Could you check a few things on this model? Use its own coordinates, in mm. A direction names the side the tool comes from. Round coordinates to 2 decimals unless told otherwise and drop trailing zeros. Loops run counter-clockwise (first coordinate to the right, second up) from the corner with the lowest first, then second, coordinate; pieces in that order, holes last. Notation, with made-up numbers: (20, 13.25) -> (51, 13.25) arc R13 cw to (51, 33.25) -> close; hole circle Ø6 at (79, 42.25). An arc over 180 degrees is marked (long way). One line per item, written item: value.
```python
from build123d import *

# Parameters (mm, degrees)
SKETCH1_R               = 3.75
BOSS_EXTRUDE1_DEPTH     = 10
SKETCH4_W               = 1
SKETCH4_H               = 1
BOSS_EXTRUDE2_DEPTH     = 2
CUT_EXTRUDE1_DEPTH      = 6.5
CUT_EXTRUDE1_DEPTH_BACK = 6.5
SKETCH5_W               = 3.094482754
SKETCH5_H               = 13.244386188
SKETCH6_R               = 3
BOSS_EXTRUDE3_DEPTH     = 6.7
SKETCH7_R               = 2.5
CUT_EXTRUDE2_DEPTH      = 1.25
FILLET2_R               = 0.25
FILLET3_R               = 0.25


with BuildPart() as part:
    # Sketch1 → Boss-Extrude1 (new body)
    with BuildSketch(Plane.XY):
        Circle(SKETCH1_R)
    extrude(amount=BOSS_EXTRUDE1_DEPTH)

    # Sketch3 → Cut-Revolve1 (revolve, cut)
    with BuildSketch(Plane(origin=(0, 0, 0), x_dir=(1, 0, 0), z_dir=(0, 1, 0)), mode=Mode.PRIVATE) as cut_revolve1_sk:
        Polygon((-3, -10), (0, -10), (0, -9), (-1, -9), align=None)
    revolve(cut_revolve1_sk.sketch.rotate(Axis((0, 0, 10), (0, 0, -1)), 180), axis=Axis((0, 0, 10), (0, 0, -1)), mode=Mode.SUBTRACT)

    # Sketch4 → Boss-Extrude2 (add)
    with BuildSketch(Plane(origin=(0, 0, 0), x_dir=(-1, 0, 0), z_dir=(0, 0, -1))):
        with Locations((0, 4)):
            Rectangle(SKETCH4_W, SKETCH4_H)
        with Locations((-4, 0)):
            Rectangle(SKETCH4_W, SKETCH4_H)
        with Locations((4, 0)):
            Rectangle(SKETCH4_W, SKETCH4_H)
        with Locations((0, -4)):
            Rectangle(SKETCH4_W, SKETCH4_H)
    extrude(amount=-BOSS_EXTRUDE2_DEPTH)

    # Sketch5 → Cut-Extrude1 (cut, two sides: drawn at the far end of the back side and taken through both)
    with BuildSketch(Plane(origin=(0, 0, 0), x_dir=(0, 0, -1), z_dir=(1, 0, 0)).offset(-CUT_EXTRUDE1_DEPTH_BACK)):
        with Locations((0.797241377, 0.144409195)):
            Rectangle(SKETCH5_W, SKETCH5_H)
    extrude(amount=CUT_EXTRUDE1_DEPTH + CUT_EXTRUDE1_DEPTH_BACK, mode=Mode.SUBTRACT)

    # Sketch6 → Boss-Extrude3 (add)
    with BuildSketch(Plane(origin=(0, 0, 0.75), x_dir=(-1, 0, 0), z_dir=(0, 0, -1))):
        with Locations(Location((0, 0, 0), (0, 0, 90))):
            Circle(SKETCH6_R)
    extrude(amount=BOSS_EXTRUDE3_DEPTH)

    # Sketch7 → Cut-Extrude2 (cut)
    with BuildSketch(Plane(origin=(0, 0, -5.95), x_dir=(-1, 0, 0), z_dir=(0, 0, -1))):
        with Locations(Location((0, 0, 0), (0, 0, 90))):
            Circle(SKETCH7_R)
    extrude(amount=-CUT_EXTRUDE2_DEPTH, mode=Mode.SUBTRACT)

    # Fillet2
    fillet2_edges = [part.edges().sort_by_distance(p)[0] for p in [
        (0, -3, -5.95),
    ]]
    fillet(fillet2_edges, radius=FILLET2_R)

    # Fillet3
    fillet3_edges = [part.edges().sort_by_distance(p)[0] for p in [
        (4.5, 0.5, 1.375),
        (4.5, -0.5, 1.375),
        (-0.5, 4.5, 1.375),
        (0.5, 4.5, 1.375),
        (-4.5, -0.5, 1.375),
        (-4.5, 0.5, 1.375),
        (0.5, -4.5, 1.375),
        (-0.5, -4.5, 1.375),
    ]]
    fillet(fillet3_edges, radius=FILLET3_R)


solid = part.part
```
Item 1: Will these pins go through, and if not, where does the flat tip stop? pin 1 Ø5 at (x, z) = (2.5, 4) entering from +Y; pin 2 Ø4.5 at (x, y) = (0, 0) entering from -Z; pin 3 Ø1 at (x, y) = (-0.5, 0.5) entering from +Z.
Output:
pin 1: stops at y = 3.75
pin 2: stops at z = -4.7
pin 3: stops at z = 9.1
Item 2: For faces 4 (the face through (3.464, -1.436, 5.31)), 5 (the face through (-2.44, -0.54, -5.33)), 6 (the face through (1, 3, 10)), which set-ups out of +Z, -Z, +X, -X, +Y, -Y let a thin tool reach every point of the face, with its end or its side?
Output:
face 4: +Z
face 5: -Z
face 6: +Z, +X, -X, +Y, -Y
Item 3: If we mould it in two halves opening along Y, with no side actions, what happens to faces 1 (the face through (0, 0, 9)), 2 (the face through (1, -3, 0.75)), 3 (the face through (0.9, 2.86, -2.43))? For each: released by +Y, released by -Y, zero draft, split by the parting line, or undercut.
Output:
face 1: undercut
face 2: zero draft
face 3: split by the parting line
Item 4: If we section it at D-D on x = -3.25: List the corners of the cut face in (y, z) for me, plus the area to 3 significant figures.
Output:
outline: (-1.87, 0.75) -> (1.87, 0.75) -> (1.87, 10) -> (-1.87, 10) -> close
area: 34.6 mm²
Item 5: If we section it at A-A on y = 0: List the corners of the cut face in (x, z) for me, plus the area to 3 significant figures.
Output:
outline: (-4.5, 0.75) -> (-3, 0.75) -> (-3, -5.7) arc R0.25 ccw to (-2.75, -5.95) -> (-2.5, -5.95) -> (-2.5, -4.7) -> (2.5, -4.7) -> (2.5, -5.95) -> (2.75, -5.95) arc R0.25 ccw to (3, -5.7) -> (3, 0.75) -> (4.5, 0.75) -> (4.5, 2) -> (3.75, 2) -> (3.75, 10) -> (3, 10) -> (1, 9) -> (-1, 9) -> (-3, 10) -> (-3.75, 10) -> (-3.75, 2) -> (-4.5, 2) -> close
area: 101 mm²
Item 6: If we section it at C-C on z = 3: List the corners of the cut face in (x, y) for me.
Output:
outline: circle Ø7.5 at (0, 0)
Item 7: I need wall thicknesses on line 1 (X direction, y = 0, z = -5.1); line 2 (Z direction, x = -3.5, y = -1); line 3 (Z direction, x = 0, y = 0). Which ranges of each line are inside material? Lowest first, please. Write a range as from..to.
Output:
line 1: x = -3..-2.5, 2.5..3
line 2: z = 0.75..10
line 3: z = -4.7..9
